Work out the finished part from the listing and answer in its coordinate system (mm). A direction names the side the tool comes from. Give positions to 0.01 mm unless a question says otherwise; leave off trailing zeros. Order: outer loops, then holes, each group sorted by start corner. A loop starts at its lowest first (then second) coordinate and runs counter-clockwise, first axis right, second up.
Autodesk Inventor part; units mm, degrees
ref_plane "YZ Plane" through (0, 0, 0) normal (1, 0, 0) x (0, 1, 0)
ref_plane "XZ Plane" through (0, 0, 0) normal (0, 1, 0) x (-1, 0, 0)
ref_plane "XY Plane" through (0, 0, 0) normal (0, 0, 1) x (1, 0, 0)
sketch "Sketch2" plane through (0, 0, 0) normal (0, 1, 0) x (-1, 0, 0)
  line L0 (-4, 4) -> (4, 4)
  line L1 (4, 4) -> (4, -4)
  line L2 (4, -4) -> (-4, -4)
  line L3 (-4, -4) -> (-4, 4)
  point P0 (0, 0)
  point P1 (0, 4)
  point P2 (-4, 0)
  dimension "d0" = 8
  dimension "d1" = 8
extrude "Extrusion1" add sketch "Sketch2" along normal blind 3.2
sketch "Sketch3" plane through (0, 0, 0) normal (0, -1, 0) x (1, 0, 0)
  line L0 (4, 4) -> (-4, 4)
  line L1 (-4, 4) -> (-4, -4)
  line L2 (-2.4, 2.4) -> (2.4, 2.4)
  line L3 (2.4, 2.4) -> (2.4, -2.4)
  line L4 (2.4, -2.4) -> (-2.4, -2.4)
  line L5 (-2.4, -2.4) -> (-2.4, 2.4)
  line L6 (-4, -4) -> (4, -4)
  line L7 (4, -4) -> (4, 4)
  line L8 (-3.6, 3.6) -> (3.6, 3.6)
  line L9 (3.6, 3.6) -> (3.6, -3.6)
  line L10 (3.6, -3.6) -> (-3.6, -3.6)
  line L11 (-3.6, -3.6) -> (-3.6, 3.6)
  point P0 (0, 0)
  point P1 (-2.4, 0)
  point P2 (0, 2.4)
  point P3 (0, 0)
  point P4 (-3.6, 0)
  point P5 (0, 3.6)
  dimension "d8" = 1.6
  dimension "d62" = 1.6
  dimension "d98" = 0.4
  dimension "d99" = 0.4
extrude "Extrusion2" cut sketch "Sketch3" against normal blind 1.6 contours L2 L3 L4 L5
extrude "Extrusion7" cut sketch "Sketch3" against normal blind 0.4 contours L7 L6 L1 L0
fillet "Fillet1" radius 0.1 8 edges at (-4, 1.8, 4) (0, 3.2, 4) (-4, 3.2, 0) (4, 1.8, 4) (4, 3.2, 0) (0, 3.2, -4) (4, 1.8, -4) (-4, 1.8, -4)
equation "\"d4\" = 0.333333 * lh"
equation "\"d8\" = d62"
equation "\"d62\" = wall"
equation "\"d98\" = gw"
equation "\"d99\" = d98"
equation "\"d11\" = 0.333333 * lh - topthk"
equation "\"d100\" = gh"
equation "\"d22\" = lf"
properties part number "3070b-DkBluishGray" material "ABS Plastic"
1. Straight lines are drawn through the part: probe 1 along Z at (x, y) = (0.75, 0.55); probe 2 along Y at (x, z) = (-2, 2). For each, find the intervals that lie inside material, in ascending order.
Findings below:
probe 1: z = -4 to -2.4, 2.4 to 4
probe 2: y = 1.6 to 3.2
2. Which of the six approach directions +Z, -Z, +X, -X, +Y, -Y give full straight-line access (tool end or side, diameter ignored) to faces 1 (the face through (-4, 2, 0)), 2 (the face through (-2.4, 1, 0))?
Findings below:
face 1: +Z, -Z, -X, +Y, -Y
face 2: -Y
3. The part is cut by section C-C (x = -1). Write down the section's boundary in (y, z).
Findings below:
outline: (0, -3.6) - (0.4, -3.6) - (0.4, -4) - (3.1, -4) arc R0.1 ccw to (3.2, -3.9) - (3.2, 3.9) arc R0.1 ccw to (3.1, 4) - (0.4, 4) - (0.4, 3.6) - (0, 3.6) - (0, 2.4) - (1.6, 2.4) - (1.6, -2.4) - (0, -2.4) - close
4. The part is cut by section A-A (y = 1.25). Write down the section's boundary in (x, z), then the cut area to 3 significant figures.
Findings below:
outline: (-4, -3.9) arc R0.1 ccw to (-3.9, -4) - (3.9, -4) arc R0.1 ccw to (4, -3.9) - (4, 3.9) arc R0.1 ccw to (3.9, 4) - (-3.9, 4) arc R0.1 ccw to (-4, 3.9) - close; hole (-2.4, -2.4) - (2.4, -2.4) - (2.4, 2.4) - (-2.4, 2.4) - close
area: 41.0 mm2
5. The mould has two halves that part along Z. Classify faces 3 (the face through (4, 2, 0)), 4 (the face through (0, 1, 2.4)), 5 (the face through (0, 2, -4)): pulls with the +Z half, pulls with the -Z half, needs draft (parallel to the pull), parting line crosses it, or undercut.
Findings below:
face 3: needs draft
face 4: undercut
face 5: pulls with the -Z half
6. Given P1, Ø4, axis at x = 1, z = 0, coming from the -Y side, flat-ended and moving along its own axis, determine where the tip first touches the part or whether it passes through.
Findings below:
P1: stops at y = 0
7. The part is cut by section B-B (z = -1). Write down the section's boundary in (x, y), then the cut area to 3 significant figures.
Findings below:
outline: (-4, 0.4) - (-3.6, 0.4) - (-3.6, 0) - (-2.4, 0) - (-2.4, 1.6) - (2.4, 1.6) - (2.4, 0) - (3.6, 0) - (3.6, 0.4) - (4, 0.4) - (4, 3.1) arc R0.1 ccw to (3.9, 3.2) - (-3.9, 3.2) arc R0.1 ccw to (-4, 3.1) - close
area: 17.6 mm2
